from build123d import *

# Parameters (mm, degrees)
SKETCH1_W           = 40
SKETCH1_H           = 40
BOSS_EXTRUDE1_DEPTH = 40
SKETCH2_W           = 20
SKETCH2_H           = 10
CUT_EXTRUDE1_DEPTH  = 40
CUT_EXTRUDE2_DEPTH  = 40
SKETCH4_W           = 20
SKETCH4_H           = 20
CUT_EXTRUDE5_DEPTH  = 40
SKETCH5_R           = 20
CUT_EXTRUDE6_DEPTH  = 30
REVOLVE1_ANGLE      = 180


with BuildPart() as part:
    # Sketch1 → Boss-Extrude1 (new body)
    with BuildSketch(Plane.XY):
        with Locations((20, 20)):
            Rectangle(SKETCH1_W, SKETCH1_H)
    extrude(amount=BOSS_EXTRUDE1_DEPTH)

    # Sketch2 → Cut-Extrude1 (cut)
    with BuildSketch(Plane.XY.offset(40)):
        with Locations((20, 5)):
            Rectangle(SKETCH2_W, SKETCH2_H)
        Polygon((0, 40), (0, 20), (20, 40), align=None)
        Polygon((20, 40), (40, 20), (40, 40), align=None)
    extrude(amount=-CUT_EXTRUDE1_DEPTH, mode=Mode.SUBTRACT)

    # Sketch3 → Cut-Extrude2 (cut)
    with BuildSketch(Plane(origin=(0, 0, 0), x_dir=(1, 0, 0), z_dir=(0, 1, 0))):
        with BuildLine():
            Line((20, 0), (0, 0))
            Line((0, 0), (0, -20))
            ThreePointArc((0, -20), (5.857864376, -5.857864376), (20, 0))
        make_face()
        with BuildLine():
            Line((40, 0), (20, 0))
            ThreePointArc((20, 0), (34.142135624, -5.857864376), (40, -20))
            Line((40, -20), (40, 0))
        make_face()
        with BuildLine():
            Line((40, -40), (40, -20))
            ThreePointArc((40, -20), (34.142135624, -34.142135624), (20, -40))
            Line((20, -40), (40, -40))
        make_face()
        with BuildLine():
            ThreePointArc((20, -40), (5.857864376, -34.142135624), (0, -20))
            Line((0, -20), (0, -40))
            Line((0, -40), (20, -40))
        make_face()
    extrude(amount=CUT_EXTRUDE2_DEPTH, mode=Mode.SUBTRACT)

    # Sketch4 → Cut-Extrude5 (cut)
    with BuildSketch(Plane(origin=(0, 0, 0), x_dir=(0, 0, -1), z_dir=(1, 0, 0))):
        Polygon((0, 40), (0, 20), (-20, 40), align=None)
        with Locations((-30, 30)):
            Rectangle(SKETCH4_W, SKETCH4_H)
    extrude(amount=CUT_EXTRUDE5_DEPTH, mode=Mode.SUBTRACT)

    # Sketch5 → Cut-Extrude6 (cut)
    with BuildSketch(Plane(origin=(0, 20, 0), x_dir=(1, 0, 0), z_dir=(0, 1, 0))):
        with Locations((20, -20)):
            Circle(SKETCH5_R)
    extrude(amount=CUT_EXTRUDE6_DEPTH, mode=Mode.SUBTRACT)

    # Sketch6 → Revolve1 (revolve)
    with BuildSketch(Plane.XY.offset(20)):
        Polygon((20, 20), (20, 40), (0, 20), align=None)
    revolve(axis=Axis((20, 20, 20), (0, -1, 0)), revolution_arc=REVOLVE1_ANGLE)


solid = part.part
The model under review builds one solid part; all positions refer to its coordinate system, in mm. A direction names the side the tool comes from. Coordinates: 2 decimals unless noted, no trailing zeros. Write each loop counter-clockwise with the first axis right and the second up, starting at its lowest first coordinate (ties: lowest second). Pieces come first, ordered by that corner, then holes. Notation, with made-up numbers: (26, 57.25) - (69, 57.25) arc R20 ccw to (69, 77.25) - close; hole circle Ø8 at (50, -26.75). An arc over 180 degrees is marked (long way). Answer as CSV lines item,"result".
(1) We need section A-A (z = 23). Give the boundary of the cut face in (x, y).
Data:
outline,"(0.23, 0) - (10, 0) - (10, 10) - (30, 10) - (30, 0) - (39.77, 0) - (39.77, 20) - (0.23, 20) - close"
(2) Tool access review of faces 1 (the flat face through (20, 20, 28)), 2 (the flat face through (10, 5, 20)), 3 (the conical face through (20, 32, 12)): name each direction out of +Z, -Z, +X, -X, +Y, -Y from which nothing blocks a thin tool from reaching the whole face with its end or side.
Data:
face 1,"+Z, +X, -X, +Y"
face 2,"+Z, -Z, -Y"
face 3,"-Z, +Y"
(3) We need section B-B (y = 33). Give the boundary of the cut face in (x, z), plus the area to 3 significant figures.
Data:
outline,"(13, 20) arc R7 ccw to (27, 20) - close"
area,"77.0 mm2"
(4) Clearance check with flat-ended pins moving along their axes: pin 1 Ø6 at (x, z) = (21.5, 22) entering from -Y; pin 2 Ø3 at (y, z) = (4.5, 18) entering from -X; pin 3 Ø22 at (x, y) = (11, 34) entering from +Z. State where each tip first meets the part, or that it passes through.
Data:
pin 1,"stops at y = 10"
pin 2,"stops at x = 0.01"
pin 3,"stops at z = 20"
(5) For line 1 along X through (y, z) = (6, 14.5); line 2 along Y through (x, z) = (19, 23); line 3 along Y through (x, z) = (6.5, 34.5), list the stretches that pass through material, from the lowest coordinate up. Write a range as [from, to].
Data:
line 1,"x = [0.77, 10], [30, 39.23]"
line 2,"y = [10, 20]"
line 3,"y = [0, 20]"
